The model under review builds one solid part; all positions refer to its coordinate system, in mm. Give positions to 0.01 mm unless a question says otherwise; leave off trailing zeros. Order: outer loops, then holes, each group sorted by start corner. A loop starts at its lowest first (then second) coordinate and runs counter-clockwise, first axis right, second up.
Autodesk Inventor part; units mm, degrees
ref_plane "YZ Plane" through (0, 0, 0) normal (1, 0, 0) x (0, 1, 0)
ref_plane "XZ Plane" through (0, 0, 0) normal (0, 1, 0) x (-1, 0, 0)
ref_plane "XY Plane" through (0, 0, 0) normal (0, 0, 1) x (1, 0, 0)
sketch "Szkic1" plane through (0, 0, 0) normal (0, 0, 1) x (1, 0, 0)
  line L0 (-2.2485, 0) -> (12.0414, 0)
  line L1 (0, -4.2485) -> (0, 24.0414)
  line L2 (10, 0) -> (1, 0)
  line L3 (0, 1) -> (0, 20)
  line L4 (2, 20) -> (2, 3)
  line L5 (3, 2) -> (10, 2)
  line L6 (0, 20) -> (2, 20)
  line L7 (10, 0) -> (10, 2)
  arc A0 (2, 3) -> (3, 2) centre (3, 3) ccw
  arc A1 (0, 1) -> (1, 0) centre (1, 1) ccw
  point P0 (0, 0)
  dimension "d0" = 20
  dimension "d1" = 10
  dimension "d2" = 2
  dimension "d3" = 1
extrude "Wyciągnięcie proste1" add sketch "Szkic1" along normal blind 300 contours A1 L1 L6 L4 A0 L5 L7 L0
sketch "Szkic2" plane through (1, 0, 0) normal (0, -1, 0) x (1, 0, 0)
  line L0 (0, 0) -> (9, 0)
  line L1 (9, 0) -> (9, 300)
  line L2 (0, 300) -> (9, 300)
  line L3 (-1, 0) -> (-1, 300)
  line L4 (-1, 300) -> (9, 290)
  line L5 (9, 290) -> (9, 300)
  line L6 (9, 300) -> (-1, 300)
  line L7 (-1, 0) -> (9, 10)
  line L8 (9, 10) -> (9, 0)
  line L9 (9, 0) -> (-1, 0)
  dimension "d6" = 135
  dimension "d7" = 45
extrude "Wyciągnięcie proste2" cut sketch "Szkic2" against normal through all contours L9 L7 L1 L0 | L6 L2 L1 L4
properties part number "kątownik_mały1" material "Aluminium 6061"
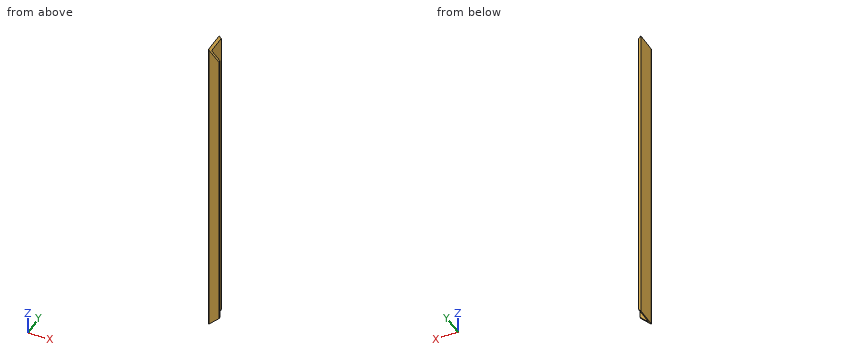
Item 1: Clearance check with a flat-ended pin moving along its axis: pin 1 Ø6 at (y, z) = (6, 88.5) entering from +X. State where the tip first meets the part, or that it passes through.
Values found:
pin 1: stops at x = 2
Item 2: For line 1 (X direction, y = 17, z = 107); line 2 (Y direction, x = 2.25, z = 197), list the stretches that pass through material, from the lowest coordinate up.
Values found:
line 1: x = 0 to 2
line 2: y = 0 to 2.34
Item 3: Take a section at B-B (y = 15.75). Give the boundary of the cut face in (x, z).
Values found:
outline: (0, 0) - (2, 2) - (2, 298) - (0, 300) - close
Item 4: Take a section at C-C (x = 6.25). Give the boundary of the cut face in (y, z).
Values found:
outline: (0, 6.25) - (2, 6.25) - (2, 293.75) - (0, 293.75) - close
Item 5: Take a section at A-A (z = 139.5). Give the boundary of the cut face in (x, y), and give its area (3 significant figures).
Values found:
outline: (0, 1) arc R1 ccw to (1, 0) - (10, 0) - (10, 2) - (3, 2) arc R1 cw to (2, 3) - (2, 20) - (0, 20) - close
area: 56.0 mm2
